```python
from build123d import *

# Parameters (mm, degrees)
SKETCH1_W                = 15.875
SKETCH1_H                = 17.4
BOSS_EXTRUDE1_DEPTH      = 6.35
M4_CLEARANCE_HOLE1_D     = 4.5
M4_CLEARANCE_HOLE1_DEPTH = 12.7
M4_CLEARANCE_HOLE1_TIP   = 1.351936393


with BuildPart() as part:
    # Sketch1 → Boss-Extrude1 (new body)
    with BuildSketch(Plane.XY):
        with Locations((-7.9375, 8.7)):
            Rectangle(SKETCH1_W, SKETCH1_H)
    extrude(amount=BOSS_EXTRUDE1_DEPTH)

    # M4 Clearance Hole1
    with Locations(Plane.XY.offset(6.35)):
        with Locations((-7.9375, 8.7)):
            Hole(M4_CLEARANCE_HOLE1_D / 2, depth=M4_CLEARANCE_HOLE1_DEPTH)
            with Locations((0, 0, -(M4_CLEARANCE_HOLE1_DEPTH + M4_CLEARANCE_HOLE1_TIP / 2))):  # 118° drill point
                Cone(0, M4_CLEARANCE_HOLE1_D / 2, M4_CLEARANCE_HOLE1_TIP, mode=Mode.SUBTRACT)


solid = part.part
```
Here's how the part is built. I have some questions about the finished solid (model axes, mm). Give positions to 0.01 mm unless a question says otherwise; leave off trailing zeros. Write each loop counter-clockwise with the first axis right and the second up, starting at its lowest first coordinate (ties: lowest second). Pieces come first, ordered by that corner, then holes.
(1) If I drill on L1, parallel to X at y = 8.75, z = 2 (3 decimals); L2, parallel to X at y = 7.25, z = 3.5 (3 decimals); L3, parallel to Y at x = -6.5, z = 1.5, over which ranges is the centre line in solid material (lowest first)?
Output values:
L1: x = -15.875 to -10.187, -5.688 to 0
L2: x = -15.875 to -9.658, -6.217 to 0
L3: y = 0 to 6.97, 10.43 to 17.4
(2) Imagine slicing it at B-B, the plane x = -7.5. Write out the boundary of the cut face in (y, z).
Output values:
outline: (0, 0) - (6.49, 0) - (6.49, 6.35) - (0, 6.35) - close; (10.91, 0) - (17.4, 0) - (17.4, 6.35) - (10.91, 6.35) - close
(3) Thinking about a two-plate mould opening in Y: for faces 1 (the face through (0, 9, 3)), 2 (the face through (-7.45, 6.504, 3.131)), 3 (the face through (-8, 0, 3)), which applies, pulls with the +Y half, pulls with the -Y half, needs draft (parallel to the pull), parting line crosses it, or undercut?
Output values:
face 1: needs draft
face 2: undercut
face 3: pulls with the -Y half
